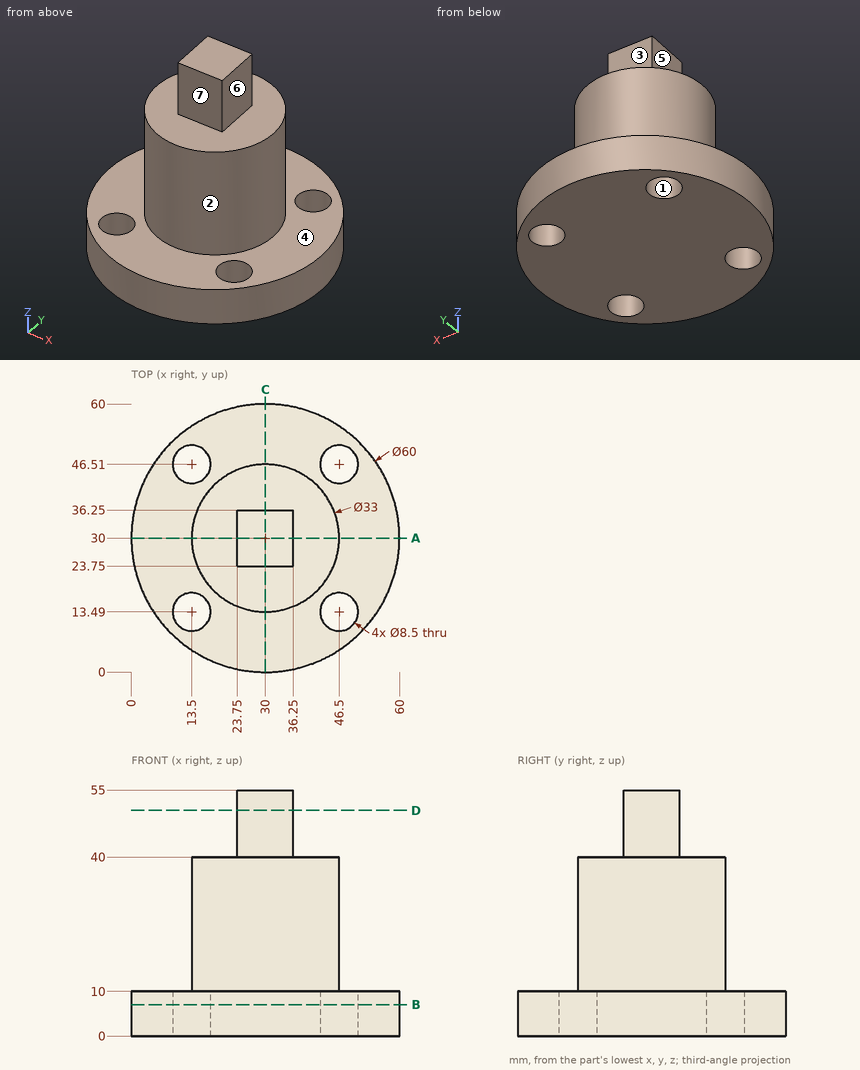
Geometry check sheet. Reference: drawing and pictorial views, mm from the part's lowest x, y, z. A direction names the side the tool comes from. Give positions to 0.01 mm unless a question says otherwise; leave off trailing zeros. Loops run counter-clockwise (first coordinate to the right, second up) from the corner with the lowest first, then second, coordinate; pieces in that order, holes last. Notation, with made-up numbers: (73, -22) - (131, -22) arc R27 cw to (131, 12) - close; hole circle Ø11 at (-4, 30.5). An arc over 180 degrees is marked (long way). One line per question, with ' | ' between items. Start each with the question number.
1. Draft check along Y on the marked faces 1, 2 and 3. Enter one of: released by +Y, released by -Y, zero draft, split by the parting line, or undercut.
2. Cross-section at A-A, the plane y = 30. Enter the section's corners in (x, z), plus the area to 3 significant figures.
3. Cross-section at B-B, the plane z = 7. Enter the section's corners in (x, y), plus the area to 3 significant figures.
4. Set-up check for the marked faces 4, 5, 6 and 7: record each of +Z, -Z, +X, -X, +Y, -Y from which the full face is reachable in a straight line by a thin tool's end or side.
5. Gauge pin test, flat ends, axial feed: pin 1 Ø4 at (y, z) = (32, 34.5) entering from +X; pin 2 Ø5 at (x, z) = (23, 27.5) entering from -Y; pin 3 Ø1.5 at (x, z) = (34.5, 32.5) entering from -Y. Record the tip position at first contact, or that the pin passes through.
6. Cross-section at D-D, the plane z = 50.5. Enter the section's corners in (x, y).
7. Material ranges on line 1 along X through (y, z) = (46, 7); line 2 along X through (y, z) = (13, 5); line 3 along Y through (x, z) = (46, 7), recorded low to high. Write a range as [from, to].
Check result:
1) face 1: undercut | face 2: split by the parting line | face 3: released by +Y
2) outline: (0, 0) - (60, 0) - (60, 10) - (46.5, 10) - (46.5, 40) - (36.25, 40) - (36.25, 55) - (23.75, 55) - (23.75, 40) - (13.5, 40) - (13.5, 10) - (0, 10) - close | area: 1,780 mm2
3) outline: circle Ø60 at (30, 30); hole circle Ø8.5 at (13.5, 13.49); hole circle Ø8.5 at (13.5, 46.51); hole circle Ø8.5 at (46.5, 13.49); hole circle Ø8.5 at (46.5, 46.51) | area: 2,600 mm2
4) face 4: +Z | face 5: +Z, -X, +Y, -Y | face 6: +Z, +X, +Y, -Y | face 7: +Z, +X, -X, -Y
5) pin 1: stops at x = 46.5 | pin 2: stops at y = 14.13 | pin 3: stops at y = 13.93
6) outline: (23.75, 23.75) - (36.25, 23.75) - (36.25, 36.25) - (23.75, 36.25) - close
7) line 1: x = [4.62, 9.28], [17.72, 42.28], [50.72, 55.38] | line 2: x = [5.28, 9.28], [17.72, 42.28], [50.72, 54.72] | line 3: y = [4.62, 9.27], [17.71, 42.29], [50.73, 55.38]
